CAD build for the part. Positions are in the model's coordinates, mm. Face numbers are marked on the shaded views. A direction names the side the tool comes from. Coordinates: 2 decimals unless noted, no trailing zeros. Order: outer loops, then holes, each group sorted by start corner. A loop starts at its lowest first (then second) coordinate and runs counter-clockwise, first axis right, second up. Notation, with made-up numbers: M 6.25,-19 L 11.25,-19 A14 ccw 11.25,3 Z; hole C 44,23 d8. An arc over 180 degrees is marked long. Write item = value, one per line.
Autodesk Inventor part; units mm, degrees
ref_plane "Work Plane1" through (0, 0, 2.5) normal (0, 0, 1) x (1, 0, 0)
ref_plane "Work Plane2" through (0, 0, -2.5) normal (0, 0, 1) x (1, 0, 0)
ref_plane "Work Plane3" through (0, 5.3975, 0) normal (0, 1, 0) x (1, 0, 0)
sketch "Sketch1" plane through (0, 0, 0) normal (0, 1, 0) x (-1, 0, 0)
  circle A0 centre (0, 0) radius 12.7
  dimension "d75" = 25.4
extrude "Extrusion1" add sketch "Sketch1" along normal blind 3.4925 and the other way blind 3.4925
ref_plane "Work Plane1" through (0, 0, 2.5) normal (0, 0, 1) x (1, 0, 0)
ref_plane "Work Plane2" through (0, 0, -2.5) normal (0, 0, 1) x (1, 0, 0)
sketch "Sketch2" plane through (0, 0, 0) normal (0, 0, 1) x (1, 0, 0)
  circle A0 centre (7.4168, 0) radius 1.7
  circle A1 centre (-7.4168, 0) radius 1.7
  point P0 (0, 0)
  dimension "d5" = 3.4
  dimension "d6" = 7.4168
  dimension "d7" = 3.4
  dimension "d8" = 7.4168
extrude "Screw hole 2" cut sketch "Sketch2" along normal blind 2.5 and the other way blind 6 contours A0
sketch "Sketch3" plane through (0, 0, 2.5) normal (0, 0, 1) x (1, 0, 0)
  circle A0 centre (7.4168, 0) radius 1.7
  circle A1 centre (7.4168, 0) radius 3.25
  point P0 (0, 0)
  dimension "d19" = 6.5
sketch "Sketch4" plane through (0, 0, -2.5) normal (0, 0, 1) x (1, 0, 0)
  circle A0 centre (7.4168, 0) radius 1.7
  circle A1 centre (7.4168, 0) radius 3.45 construction
  line L0 (7.4168, -3.45) -> (4.429, -1.725)
  line L1 (4.429, -1.725) -> (4.429, 6.985)
  line L2 (10.4046, 6.985) -> (10.4046, -1.725)
  line L3 (10.4046, -1.725) -> (7.4168, -3.45)
  line L4 (10.4046, 6.985) -> (4.429, 6.985)
  point P0 (0, 0)
  dimension "d22" = 6.9
sketch "Sketch5" plane through (0, 0, -2.5) normal (0, 0, 1) x (1, 0, 0)
  circle A0 centre (-7.422, 0) radius 3.25
  point P0 (0, 0)
  dimension "d25" = 6.5
extrude "Access Hole 1" cut sketch "Sketch5" against normal through all
extrude "Access Hole 2" cut sketch "Sketch3" along normal through all contours A0 | A1
extrude "Nut well 2" cut sketch "Sketch4" against normal blind 2.794 contours A0 | L0 L1 L4 L2 L3
sketch "Sketch7" plane through (0, 0, 2.5) normal (0, 0, 1) x (1, 0, 0)
  circle A0 centre (-7.422, 0) radius 3.25 construction
  circle A1 centre (-7.422, 0) radius 3.45 construction
  line L0 (-7.422, -3.25) -> (-10.2365, -1.625)
  line L1 (-10.2365, -1.625) -> (-10.2365, 5.3975)
  line L2 (-4.6074, 5.3975) -> (-4.6074, -1.625)
  line L3 (-4.6074, -1.625) -> (-7.422, -3.25)
  line L4 (16.6201, 5.3975) -> (-16.6201, 5.3975)
  line L5 (-10.2365, 5.3975) -> (-4.6074, 5.3975)
  point P0 (0, 0)
  dimension "d48" = 6.9
extrude "Nut Well 1" cut sketch "Sketch7" along normal blind 2.794
sketch "Sketch8" plane through (0, 0, 0) normal (0, 0, 1) x (1, 0, 0)
  circle A0 centre (-7.422, 0) radius 3.25
  circle A1 centre (-7.422, 0) radius 1.7
  point P0 (0, 0)
  dimension "d51" = 3.4
extrude "Screw Hole 1" cut sketch "Sketch8" along normal blind 6 and the other way blind 2.5 contours A1
ref_plane "Work Plane3" through (0, 5.3975, 0) normal (0, 1, 0) x (1, 0, 0)
sketch "Sketch9" plane through (0, 5.3975, 0) normal (0, 1, 0) x (1, 0, 0)
  arc A0 (1.9431, -2.5908) -> (-1.9431, -2.5908) centre (0, 0) ccw
  line L0 (-1.9431, -2.5908) -> (1.9431, -2.5908)
  dimension "d56" = 6.477
  dimension "d57" = 2.5908
extrude "Center shaft" cut sketch "Sketch9" against normal through all
ref_plane "Work Plane4" through (0, 5.3975, 0) normal (0, 1, 0) x (1, 0, 0)
sketch "Sketch10" plane through (0, 5.3975, 0) normal (0, 1, 0) x (1, 0, 0)
  circle A0 centre (0, 9.779) radius 1.9304
  circle A1 centre (0, -9.779) radius 1.9304
  point P0 (0, 0)
  point P1 (0, -8.001)
  dimension "d60" = 3.8608
  dimension "d61" = 9.779
  dimension "d62" = 3.8608
  dimension "d63" = 9.779
extrude "Wheel holes" cut sketch "Sketch10" against normal through all
split "Split1" plane through (0, 0, 0) removes the side toward (0, 0, 1)
properties part number "clamping hub .770 .25 D bore right"
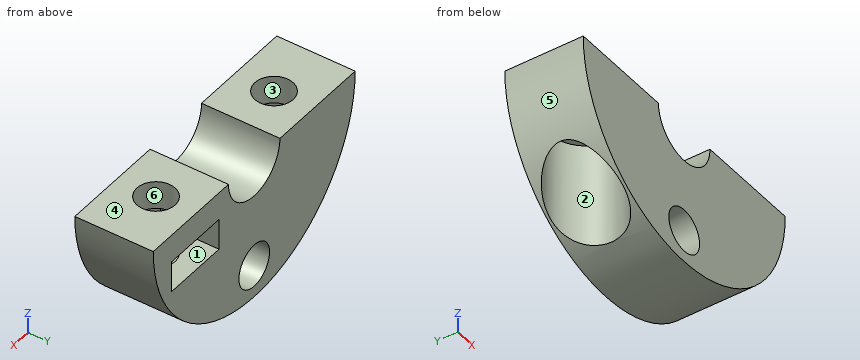
(1) Pin check, flat tips, straight feed: pin 1 Ø3 at (x, y) = (8, -1.5) entering from -Z; pin 2 Ø1.7 at (x, y) = (6.5, -0.5) entering from +Z; pin 3 Ø2 at (x, y) = (7.42, 0) entering from +Z; pin 4 Ø0.8 at (y, z) = (1.5, -3.5) entering from +X. Stop position of each tip, or through.
Evaluation:
pin_1 = -10.91
pin_2 = 0
pin_3 = -6
pin_4 = 12.32
(2) Pull direction X, two halves, no side cores. Call the marked faces 4, 5 and 6: +X half, -X half, draft (parallel to the pull), parting line (faces both ways), or undercut.
Evaluation:
face_4 = draft
face_5 = parting line
face_6 = undercut
(3) Slice it at B-B, the plane y = 0.25. Write the cut outline in (x, z).
Evaluation:
outline = M -12.7,0 A12.7 ccw -10.66,-6.9 L -10.66,-2.5 L -9.1,-2.5 L -9.1,0 Z; M -5.74,-2.5 L -4.18,-2.5 L -4.18,-11.99 A12.7 ccw 12.7,0 L 9.1,0 L 9.1,-2.5 L 10.4,-2.5 L 10.4,-5.29 L 9.1,-5.29 L 9.1,-6 L 5.74,-6 L 5.74,-5.29 L 4.43,-5.29 L 4.43,-2.5 L 5.74,-2.5 L 5.74,0 L 3.24,0 A3.24 cw -3.24,0 L -5.74,0 Z; hole C 0,-9.78 d3.86
(4) Slice it at D-D, the plane z = -9. Write the cut outline in (x, y).
Evaluation:
outline = M -8.96,-3.49 L -1.77,-3.49 L -1.77,3.49 L -8.96,3.49 L -8.96,2.86 A3.25 cw long -8.96,-2.86 Z; M 1.77,-3.49 L 8.96,-3.49 L 8.96,3.49 L 1.77,3.49 Z
(5) Slice it at C-C, the plane z = -3. State how many separate pieces and enclosed holes the cut face has, then the cut area to 3 significant figures.
Evaluation:
separate_pieces = 2
enclosed_holes = 1
area = 85.8 mm²
(6) Wall check: line 1 (X direction, y = 0, z = -5.5); line 2 (X direction, y = -3, z = -4.5); line 3 (X direction, y = 1, z = -1.5). Give the ranges that are in metal, low to high. Write a range as from..to.
Evaluation:
line_1 = -11.45..-10.67, -4.17..5.72, 9.12..11.45
line_2 = -11.88..-8.67, -6.17..6.64, 8.2..11.88
line_3 = -12.61..-8.8, -6.05..-2.87, 2.87..6.04, 8.79..12.61
(7) Tool access for the marked faces 1, 2 and 3: list every direction of +Z, -Z, +X, -X, +Y, -Y with a clear straight run to the whole face (end or side of a thin tool).
Evaluation:
face_1 = +Y
face_2 = -Z
face_3 = +Z, -Z
(8) Slice it at A-A, the plane x = 0. Write the cut outline in (y, z), then the cut area to 3 significant figures.
Evaluation:
outline = M -3.49,-12.7 L 3.49,-12.7 L 3.49,-11.71 L -3.49,-11.71 Z; M -3.49,-7.85 L 3.49,-7.85 L 3.49,-3.24 L -3.49,-3.24 Z
area = 39.1 mm²
